from build123d import *

# Parameters (mm, degrees)
F0_R     = 9.2075
F1_DEPTH = 9.525
F2_R     = 11.43
F3_DEPTH = 2.54
F4_W     = 2.54
F4_H     = 1.016
F5_DEPTH = 2.5
F6_R     = 1


with BuildPart() as f1:
    # F0 (on Top) → F1 (new body)
    with BuildSketch(Plane.XY):
        Circle(F0_R)
        with BuildLine():
            ThreePointArc((-4.7279164178, 4.7013149858), (2.5428501267, 6.1635598061), (6.6675, 0))
            ThreePointArc((6.6675, 0), (6.6092244332, -0.8796070953), (6.4354164178, -1.7438382319))
            ThreePointArc((6.4354164178, -1.7438382319), (6.3636547335, -1.9898378534), (6.2824932589, -2.2328982741))
            ThreePointArc((6.2824932589, -2.2328982741), (-3.33375, -5.7742243797), (-5.0749932589, 4.3243496242))
            ThreePointArc((-5.0749932589, 4.3243496242), (-4.9050774972, 4.5161677335), (-4.7279164178, 4.7013149858))
        make_face(mode=Mode.SUBTRACT)
        with BuildLine():
            Line((6.4354164178, -1.7438382319), (-4.7279164178, 4.7013149858))
            ThreePointArc((-4.7279164178, 4.7013149858), (-4.9050774972, 4.5161677335), (-5.0749932589, 4.3243496242))
            Line((-5.0749932589, 4.3243496242), (6.2824932589, -2.2328982741))
            ThreePointArc((6.2824932589, -2.2328982741), (6.3636547335, -1.9898378534), (6.4354164178, -1.7438382319))
        make_face()
    extrude(amount=F1_DEPTH)

    # F2 (on face) → F3 (join)
    with BuildSketch(Plane.XY.offset(9.525)):
        Circle(F2_R)
        with BuildLine():
            ThreePointArc((-4.7279164178, 4.7013149858), (3.33375, 5.7742243797), (6.4354164178, -1.7438382319))
            Line((6.4354164178, -1.7438382319), (-4.7279164178, 4.7013149858))
        make_face(mode=Mode.SUBTRACT)
    extrude(amount=F3_DEPTH)

    # F4 (on face) → F5 (join)
    with BuildSketch(Plane(origin=(0, 0, 9.525), x_dir=(1, 0, 0), z_dir=(0, 0, -1))):
        with Locations((0, -9.6274932014)):
            Rectangle(F4_W, F4_H)
    extrude(amount=F5_DEPTH)

    # F6
    f6_edges = [f1.edges().sort_by_distance(p)[0] for p in [
        (-4.727916, 4.701315, 6.0325),
        (6.435416, -1.743838, 6.0325),
        (-5.074993, 4.32435, 4.7625),
        (6.282493, -2.232898, 4.7625),
    ]]
    fillet(f6_edges, radius=F6_R)


solid = f1.part
Work out the finished part from the listing and answer in its coordinate system (mm). A direction names the side the tool comes from. Give positions to 0.01 mm unless a question says otherwise; leave off trailing zeros. Order: outer loops, then holes, each group sorted by start corner. A loop starts at its lowest first (then second) coordinate and runs counter-clockwise, first axis right, second up. Notation, with made-up numbers: (20, 67) -> (55, 67) arc R32 ccw to (55, 95) -> close; hole circle Ø2 at (-14, 50.25). An arc over 180 degrees is marked (long way). Answer as a JSON object with one key per item and string values. Group by question number.
1. Flat-ended cylindrical pins translate along their axes: pin 1 Ø0.5 at (y, z) = (9.5, 8.5) entering from -X; pin 2 Ø6 at (x, z) = (-6.5, 2) entering from -Y; pin 3 Ø4 at (y, z) = (1, 2.5) entering from +X. Find the tip coordinate at first contact, or state that the pin passes through.
2. The mould has two halves that part along Y. Classify faces 1 (the cylindrical face through (10.902, 3.433, 10.777)), 2 (the cylindrical face through (5.973, -2.386, 4.829)), 3 (the flat face through (0, 9.6, 7.025)): released by +Y, released by -Y, zero draft, split by the parting line, or undercut.
3. A tool of negligible diameter and unlimited length cuts with its end or side. For faces 4 (the cylindrical face through (-3.958, 4.807, 6.117)), 5 (the cylindrical face through (-3.2, -5.85, 4.7)), 6 (the flat face through (0, 10.135, 8)), 7 (the flat face through (1.27, 9.6, 8.3)), 8 (the flat face through (-1.27, 9.6, 8.3)), from which of +Z, -Z, +X, -X, +Y, -Y can it reach the whole face along a straight path? Write none if from no direction.
4. Section A-A on z = 10.75 is taken. Determine the outline of the cut face in (x, y) (1 decimal), plus the area to 3 significant figures.
5. Section C-C on z = 8 is taken. Determine the outline of the cut face in (x, y) (1 decimal).
6. Consider line 1 along X through (y, z) = (3.25, 3.5); line 2 along Y through (x, z) = (1, 3.25); line 3 along Y through (x, z) = (-2.5, 5.25). Determine where each line is inside the solid, lowest interval first. Write a range as [from, to].
7. Section D-D on x = 8.5 is taken. Determine the outline of the cut face in (y, z) (1 decimal).
8. Section B-B on x = 0 is taken. Determine the outline of the cut face in (y, z) (1 decimal).
Result sheet:
{
 "1": {"pin 1": "stops at x = -1.27", "pin 2": "stops at y = -8.52", "pin 3": "stops at x = 9.21"},
 "2": {"face 1": "split by the parting line", "face 2": "undercut", "face 3": "zero draft"},
 "3": {"face 4": "+Z, -Z", "face 5": "-Z", "face 6": "-Z, +X, -X, +Y", "face 7": "-Z, +X, +Y", "face 8": "-Z, -X, +Y"},
 "4": {"outline": "circle Ø22.9 at (0, 0); hole (-3.5, 4) -> (5.2, -1) arc R1 ccw to (6.7, -0.2) arc R6.7 ccw to (-3.5, 5.7) arc R1 ccw to start", "area": "364 mm^2"},
 "5": {"outline": "(-1.3, 9.1) arc R9.2 ccw (long way) to (1.3, 9.1) -> (1.3, 10.1) -> (-1.3, 10.1) -> close; hole (-5.6, 3.5) arc R6.7 ccw (long way) to (5.9, -3.1) arc R1 ccw to (5.5, -1.8) -> (-4.3, 3.9) arc R1 ccw to start; hole (-3.5, 4) -> (5.2, -1) arc R1 ccw to (6.7, -0.2) arc R6.7 ccw to (-3.5, 5.7) arc R1 ccw to start"},
 "6": {"line 1": "x = [-8.61, -5.82], [-3.21, -2.21], [5.82, 8.61]", "line 2": "y = [-9.15, -6.59], [0.82, 1.39], [6.59, 9.15]", "line 3": "y = [-8.86, -6.18], [2.84, 3.42], [6.18, 8.86]"},
 "7": {"outline": "(-7.6, 9.5) -> (-3.5, 9.5) -> (-3.5, 0) -> (3.5, 0) -> (3.5, 9.5) -> (7.6, 9.5) -> (7.6, 12.1) -> (-7.6, 12.1) -> close"},
 "8": {"outline": "(-11.4, 9.5) -> (-9.2, 9.5) -> (-9.2, 0) -> (-6.7, 0) -> (-6.7, 9.5) -> (1.4, 9.5) -> (1.4, 0) -> (2, 0) -> (2, 12.1) -> (-11.4, 12.1) -> close; (6.7, 0) -> (9.2, 0) -> (9.2, 7) -> (10.1, 7) -> (10.1, 9.5) -> (11.4, 9.5) -> (11.4, 12.1) -> (6.7, 12.1) -> close"}
}
